CAD build for the part. Positions are in the model's coordinates, mm. Face numbers are marked on the shaded views. A direction names the side the tool comes from. Round coordinates to 2 decimals unless told otherwise and drop trailing zeros. Write each loop counter-clockwise with the first axis right and the second up, starting at its lowest first coordinate (ties: lowest second). Pieces come first, ordered by that corner, then holes. Notation, with made-up numbers: (-22.5, -28) - (20.5, -28) arc R21 cw to (20.5, -7) - close; hole circle Ø7 at (-19, 37.5). An arc over 180 degrees is marked (long way). Put each result on its own line as item: value. Start each with the question number.
Item 1: Pin check, flat tips, straight feed: pin 1 Ø0.8 at (y, z) = (0, 0) entering from -X; pin 2 Ø1.5 at (x, y) = (-5, 5.5) entering from -Z; pin 3 Ø8 at (y, z) = (-3.5, 5) entering from +X; pin 4 Ø10 at (y, z) = (3.5, 3) entering from -X. Stop position of each tip, or through.
Item 2: Drill centre lines: line 1 (Z direction, x = -14, y = 0); line 2 (Z direction, x = -22.75, y = 0); line 3 (Y direction, x = 20.5, z = -3.5). Where is each one in solid material? Low to high. Write a range as from..to.
Item 3: 3-axis set-ups, long thin cutter, end or side, ignore diameter. For the marked faces 1 and 2: which of +Z, -Z, +X, -X, +Y, -Y reach the whole face in a straight line?
Item 4: Cut at A-A (x = -3). Give the cut face in (y, z), and give its area (3 significant figures).
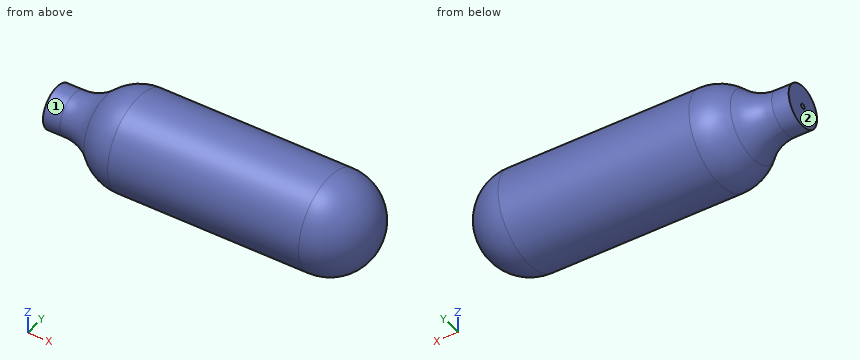
```python
from build123d import *

# Parameters (mm, degrees)
F2_R     = 9.398
F4_R     = 9.398
F5_R     = 0.508
F6_DEPTH = 25.4


# Not quite as in the source:
# - a fillet or chamfer that OpenCascade refuses, or shapes differently, is made with other operations: its cross-section is extruded or revolved along the edge and cut away or added


with BuildPart() as f1:
    # F0 (on Front) → F1 (revolve)
    with BuildSketch(Plane.XZ):
        Polygon((-31.5141436086, 0), (0, 0), (32.4938563914, 0), (32.4938563914, 9.4996), (-23.5131436086, 9.4996), (-23.5131436086, 4.2418), (-31.5141436086, 4.2418), align=None)
    revolve(axis=Axis((16.2469281957, 0, 0), (1, 0, 0)))

    # F2
    f2_edges = [f1.edges().sort_by_distance(p)[0] for p in [
        (32.493856, 0, -9.4996),
    ]]
    fillet(f2_edges, radius=F2_R)

    # F3: fillet of radius 9.398 on 1 edges, made by hand

    # F3_s1 → F3_t2 (revolve, cut)
    with BuildSketch(Plane.XZ):
        with BuildLine():
            ThreePointArc((-15.0762515291, 9.4996), (-20.0468050396, 8.0775640044), (-23.5131436086, 4.2418))
            Line((-23.5131436086, 4.2418), (-23.5131436086, 9.4996))
            Line((-23.5131436086, 9.4996), (-15.0762515291, 9.4996))
        make_face()
    revolve(axis=Axis((-23.5131436086, 0, 0), (1, 0, 0)), mode=Mode.SUBTRACT)

    # F4
    f4_edges = [f1.edges().sort_by_distance(p)[0] for p in [
        (-23.513144, 0, -4.2418),
    ]]
    fillet(f4_edges, radius=F4_R)

    # F5 (on face) → F6 (cut)
    with BuildSketch(Plane(origin=(-31.5141436086, 0, 0), x_dir=(0, -1, 0), z_dir=(-1, 0, 0))):
        Circle(F5_R)
    extrude(amount=-F6_DEPTH, mode=Mode.SUBTRACT)


solid = f1.part
```
Output values:
1. pin 1: x = -6.11
1. pin 2: z = -8.23
1. pin 3: x = 32.28
1. pin 4: x = -31.51
2. line 1: -9.5..-0.51, 0.51..9.5
2. line 2: -5.92..-0.51, 0.51..5.92
2. line 3: -8.83..8.83
3. face 1: -X
3. face 2: +Z, -Z, -X, +Y, -Y
4. outline: circle Ø19 at (0, 0)
4. area: 284 mm2
